Design review of the part built by this model. Coordinates are the model's own, in mm. A direction names the side the tool comes from. Give positions to 0.01 mm unless a question says otherwise; leave off trailing zeros. Write each loop counter-clockwise with the first axis right and the second up, starting at its lowest first coordinate (ties: lowest second). Pieces come first, ordered by that corner, then holes. Notation, with made-up numbers: (-11, 30.5) -> (19, 30.5) arc R34 ccw to (19, 61.5) -> close; hole circle Ø10 at (7, -30). An arc over 180 degrees is marked (long way). Write each question's results on one line, items separated by ' | '. Start each with the question number.
(1) Clearance check with a flat-ended pin moving along its axis: pin 1 (3.5 mm diameter, centred on x = -88.5, z = 0, fed in from +Y). State where the tip first meets the part, or that it passes through.
(2) Take a section at C-C (y = 1.15). Count the separate pieces of the cut face and the enclosed holes in it, plus the area to 3 significant figures.
(3) Take a section at B-B (z = -66.5). State the section outline as (x, y) points.
(4) For faces 4 (the face through (0.594, 0.74, -76.204)), 5 (the face through (50.105, 0.74, 29.214)), list the 3-axis set-ups (+Z, -Z, +X, -X, +Y, -Y) from which the entire face can be reached by the end or side of a thin tool; tool diameter is ignored.
(5) Take a section at A-A (z = 36.5). State the section outline as (x, y) points, plus the area to 3 significant figures.
(6) To check wall thickness, follow probe 1 along X at (y, z) = (0.25, -43.5); probe 2 along Z at (x, y) = (-42, 1.4); probe 3 along Z at (x, y) = (-5.5, 0.45). State the ranges of each line that lie inside material, in increasing order.
(7) Mouldability with a two-part tool opening along X and no side actions: class faces 1 (the face through (-42.715, 0.74, 51.984)), 2 (the face through (-15, 1.5, -46)), 3 (the face through (-66.29, 0.74, 37.59)) as released by +X, released by -X, zero draft, split by the parting line, or undercut.
from build123d import *

# Parameters (mm, degrees)
EXTRUDE_1_DEPTH = 1.5


with BuildPart() as part:
    # Эскиз1 → Бобышка-Вытянуть1 (new body)
    with BuildSketch(Plane(origin=(0, 0, 0), x_dir=(1, 0, 0), z_dir=(0, 1, 0))):
        with BuildLine():
            Line((-40.022758664, 88.321451465), (-48.25, 83.571451465))
            Line((-48.25, 83.571451465), (-56.477241336, 78.821451465))
            ThreePointArc((-56.477241336, 78.821451465), (-65.99206702, 38.100537658), (-96.5, 9.5))
            Line((-96.5, 9.5), (-96.5, 0))
            Line((-96.5, 0), (-96.5, -9.5))
            ThreePointArc((-96.5, -9.5), (-65.99206702, -38.100537658), (-56.477241336, -78.821451465))
            Line((-56.477241336, -78.821451465), (-48.25, -83.571451465))
            Line((-48.25, -83.571451465), (-40.022758664, -88.321451465))
            ThreePointArc((-40.022758664, -88.321451465), (0, -76.201075317), (40.022758664, -88.321451465))
            Line((40.022758664, -88.321451465), (48.25, -83.571451465))
            Line((48.25, -83.571451465), (56.477241336, -78.821451465))
            ThreePointArc((56.477241336, -78.821451465), (65.99206702, -38.100537658), (96.5, -9.5))
            Line((96.5, -9.5), (96.5, 0))
            Line((96.5, 0), (96.5, 9.5))
            ThreePointArc((96.5, 9.5), (65.99206702, 38.100537658), (56.477241336, 78.821451465))
            Line((56.477241336, 78.821451465), (48.25, 83.571451465))
            Line((48.25, 83.571451465), (40.022758664, 88.321451465))
            ThreePointArc((40.022758664, 88.321451465), (0, 76.201075317), (-40.022758664, 88.321451465))
        make_face()
        with BuildLine():
            Line((27.673728715, 69.932304169), (19.76108985, 56.227211632))
            ThreePointArc((19.76108985, 56.227211632), (18.754131872, 55.363280199), (17.428071074, 55.319637911))
            ThreePointArc((17.428071074, 55.319637911), (0, 58), (-17.428071074, 55.319637911))
            ThreePointArc((-17.428071074, 55.319637911), (-18.754131872, 55.363280199), (-19.76108985, 56.227211632))
            Line((-19.76108985, 56.227211632), (-27.673728715, 69.932304169))
            ThreePointArc((-27.673728715, 69.932304169), (-27.490161024, 72.198084576), (-25.306162986, 72.828648227))
            ThreePointArc((-25.306162986, 72.828648227), (0, 68.701075317), (25.306162986, 72.828648227))
            ThreePointArc((25.306162986, 72.828648227), (27.490161024, 72.198084576), (27.673728715, 69.932304169))
        make_face(mode=Mode.SUBTRACT)
        with BuildLine():
            Line((-46.726287598, 58.932304169), (-38.813648733, 45.227211632))
            ThreePointArc((-38.813648733, 45.227211632), (-38.568941153, 43.923194727), (-39.194176222, 42.752971245))
            ThreePointArc((-39.194176222, 42.752971245), (-50.229473419, 29), (-56.622247296, 12.566666667))
            ThreePointArc((-56.622247296, 12.566666667), (-57.323073025, 11.440085472), (-58.574738582, 11))
            Line((-58.574738582, 11), (-74.400016313, 11))
            ThreePointArc((-74.400016313, 11), (-76.270455859, 12.291864487), (-75.724540981, 14.498544095))
            ThreePointArc((-75.724540981, 14.498544095), (-59.496876492, 34.350537658), (-50.418377995, 58.330104132))
            ThreePointArc((-50.418377995, 58.330104132), (-48.780294835, 59.906220089), (-46.726287598, 58.932304169))
        make_face(mode=Mode.SUBTRACT)
        with BuildLine():
            Line((74.400016313, 11), (58.574738582, 11))
            ThreePointArc((58.574738582, 11), (57.323073025, 11.440085472), (56.622247296, 12.566666667))
            ThreePointArc((56.622247296, 12.566666667), (50.229473419, 29), (39.194176222, 42.752971245))
            ThreePointArc((39.194176222, 42.752971245), (38.568941153, 43.923194727), (38.813648733, 45.227211632))
            Line((38.813648733, 45.227211632), (46.726287598, 58.932304169))
            ThreePointArc((46.726287598, 58.932304169), (48.780294835, 59.906220089), (50.418377995, 58.330104132))
            ThreePointArc((50.418377995, 58.330104132), (59.496876492, 34.350537658), (75.724540981, 14.498544095))
            ThreePointArc((75.724540981, 14.498544095), (76.270455859, 12.291864487), (74.400016313, 11))
        make_face(mode=Mode.SUBTRACT)
        with BuildLine():
            Line((46.726287598, -58.932304169), (38.813648733, -45.227211632))
            ThreePointArc((38.813648733, -45.227211632), (38.568941153, -43.923194727), (39.194176222, -42.752971245))
            ThreePointArc((39.194176222, -42.752971245), (50.229473419, -29), (56.622247296, -12.566666667))
            ThreePointArc((56.622247296, -12.566666667), (57.323073025, -11.440085472), (58.574738582, -11))
            Line((58.574738582, -11), (74.400016313, -11))
            ThreePointArc((74.400016313, -11), (76.270455859, -12.291864487), (75.724540981, -14.498544095))
            ThreePointArc((75.724540981, -14.498544095), (59.496876492, -34.350537658), (50.418377995, -58.330104132))
            ThreePointArc((50.418377995, -58.330104132), (48.780294835, -59.906220089), (46.726287598, -58.932304169))
        make_face(mode=Mode.SUBTRACT)
        with BuildLine():
            Line((-27.673728715, -69.932304169), (-19.76108985, -56.227211632))
            ThreePointArc((-19.76108985, -56.227211632), (-18.754131872, -55.363280199), (-17.428071074, -55.319637911))
            ThreePointArc((-17.428071074, -55.319637911), (0, -58), (17.428071074, -55.319637911))
            ThreePointArc((17.428071074, -55.319637911), (18.754131872, -55.363280199), (19.76108985, -56.227211632))
            Line((19.76108985, -56.227211632), (27.673728715, -69.932304169))
            ThreePointArc((27.673728715, -69.932304169), (27.490161024, -72.198084576), (25.306162986, -72.828648227))
            ThreePointArc((25.306162986, -72.828648227), (0, -68.701075317), (-25.306162986, -72.828648227))
            ThreePointArc((-25.306162986, -72.828648227), (-27.490161024, -72.198084576), (-27.673728715, -69.932304169))
        make_face(mode=Mode.SUBTRACT)
        with BuildLine():
            Line((-74.400016313, -11), (-58.574738582, -11))
            ThreePointArc((-58.574738582, -11), (-57.323073025, -11.440085472), (-56.622247296, -12.566666667))
            ThreePointArc((-56.622247296, -12.566666667), (-50.229473419, -29), (-39.194176222, -42.752971245))
            ThreePointArc((-39.194176222, -42.752971245), (-38.568941153, -43.923194727), (-38.813648733, -45.227211632))
            Line((-38.813648733, -45.227211632), (-46.726287598, -58.932304169))
            ThreePointArc((-46.726287598, -58.932304169), (-48.780294835, -59.906220089), (-50.418377995, -58.330104132))
            ThreePointArc((-50.418377995, -58.330104132), (-59.496876492, -34.350537658), (-75.724540981, -14.498544095))
            ThreePointArc((-75.724540981, -14.498544095), (-76.270455859, -12.291864487), (-74.400016313, -11))
        make_face(mode=Mode.SUBTRACT)
        with BuildLine():
            ThreePointArc((-23.75, 41.13620668), (-41.13620668, 23.75), (-47.5, 0))
            ThreePointArc((-47.5, 0), (-41.13620668, -23.75), (-23.75, -41.13620668))
            ThreePointArc((-23.75, -41.13620668), (0, -47.5), (23.75, -41.13620668))
            ThreePointArc((23.75, -41.13620668), (41.13620668, -23.75), (47.5, 0))
            ThreePointArc((47.5, 0), (41.13620668, 23.75), (23.75, 41.13620668))
            ThreePointArc((23.75, 41.13620668), (0, 47.5), (-23.75, 41.13620668))
        make_face(mode=Mode.SUBTRACT)
        with BuildLine():
            ThreePointArc((-87, 0), (-88.5, 1.5), (-90, 0))
            ThreePointArc((-90, 0), (-88.5, -1.5), (-87, 0))
        make_face(mode=Mode.SUBTRACT)
        with BuildLine():
            ThreePointArc((-62, 0), (-63.5, 1.5), (-65, 0))
            ThreePointArc((-65, 0), (-63.5, -1.5), (-62, 0))
        make_face(mode=Mode.SUBTRACT)
        with BuildLine():
            ThreePointArc((-32.5, 56.291651246), (-33.049038106, 54.24261314), (-31, 53.693575035))
            ThreePointArc((-31, 53.693575035), (-30.450961894, 55.74261314), (-32.5, 56.291651246))
        make_face(mode=Mode.SUBTRACT)
        with BuildLine():
            ThreePointArc((-45, 77.942286341), (-45.549038106, 75.893248235), (-43.5, 75.344210129))
            ThreePointArc((-43.5, 75.344210129), (-42.950961894, 77.393248235), (-45, 77.942286341))
        make_face(mode=Mode.SUBTRACT)
        with BuildLine():
            ThreePointArc((32.5, 56.291651246), (30.450961894, 55.74261314), (31, 53.693575035))
            ThreePointArc((31, 53.693575035), (33.049038106, 54.24261314), (32.5, 56.291651246))
        make_face(mode=Mode.SUBTRACT)
        with BuildLine():
            ThreePointArc((45, 77.942286341), (42.950961894, 77.393248235), (43.5, 75.344210129))
            ThreePointArc((43.5, 75.344210129), (45.549038106, 75.893248235), (45, 77.942286341))
        make_face(mode=Mode.SUBTRACT)
        with BuildLine():
            ThreePointArc((65, 0), (63.5, 1.5), (62, 0))
            ThreePointArc((62, 0), (63.5, -1.5), (65, 0))
        make_face(mode=Mode.SUBTRACT)
        with BuildLine():
            ThreePointArc((90, 0), (88.5, 1.5), (87, 0))
            ThreePointArc((87, 0), (88.5, -1.5), (90, 0))
        make_face(mode=Mode.SUBTRACT)
        with BuildLine():
            ThreePointArc((32.5, -56.291651246), (33.049038106, -54.24261314), (31, -53.693575035))
            ThreePointArc((31, -53.693575035), (30.450961894, -55.74261314), (32.5, -56.291651246))
        make_face(mode=Mode.SUBTRACT)
        with BuildLine():
            ThreePointArc((45, -77.942286341), (45.549038106, -75.893248235), (43.5, -75.344210129))
            ThreePointArc((43.5, -75.344210129), (42.950961894, -77.393248235), (45, -77.942286341))
        make_face(mode=Mode.SUBTRACT)
        with BuildLine():
            ThreePointArc((-32.5, -56.291651246), (-30.450961894, -55.74261314), (-31, -53.693575035))
            ThreePointArc((-31, -53.693575035), (-33.049038106, -54.24261314), (-32.5, -56.291651246))
        make_face(mode=Mode.SUBTRACT)
        with BuildLine():
            ThreePointArc((-45, -77.942286341), (-42.950961894, -77.393248235), (-43.5, -75.344210129))
            ThreePointArc((-43.5, -75.344210129), (-45.549038106, -75.893248235), (-45, -77.942286341))
        make_face(mode=Mode.SUBTRACT)
    extrude(amount=EXTRUDE_1_DEPTH)


solid = part.part
Report:
1) pin 1: y = 1.5
2) separate pieces: 1 | enclosed holes: 19 | area: 11,700 mm2
3) outline: (-56.74, 0) -> (-25.69, 0) -> (-25.69, 1.5) -> (-56.74, 1.5) -> close; (25.69, 0) -> (56.74, 0) -> (56.74, 1.5) -> (25.69, 1.5) -> close
4) face 4: -Z, +Y, -Y | face 5: +Y, -Y
5) outline: (-66.94, 0) -> (-58.3, 0) -> (-58.3, 1.5) -> (-66.94, 1.5) -> close; (-45.07, 0) -> (-30.4, 0) -> (-30.4, 1.5) -> (-45.07, 1.5) -> close; (30.4, 0) -> (45.07, 0) -> (45.07, 1.5) -> (30.4, 1.5) -> close; (58.3, 0) -> (66.94, 0) -> (66.94, 1.5) -> (58.3, 1.5) -> close | area: 70.0 mm2
6) probe 1: -63.17 to -54.97, -38.68 to -19.08, 19.08 to 38.68, 54.97 to 63.17 | probe 2: -87.18 to -50.75, -40 to -22.19, 22.19 to 40, 50.75 to 87.18 | probe 3: -76.41 to -68.89, -57.74 to -47.18, 47.18 to 57.74, 68.89 to 76.41
7) face 1: undercut | face 2: zero draft | face 3: released by -X
